from build123d import *

# Parameters (mm, degrees)
BOSS_EXTRUDE1_START            = -6.5
BOSS_EXTRUDE1_OUTLINE_W        = 7.364142843
BOSS_EXTRUDE1_OUTLINE_H        = 4.764142843
BOSS_EXTRUDE1_DEPTH            = 6.5
SKETCH2_W                      = 7.364142843
SKETCH2_H                      = 6.5
BOSS_EXTRUDE2_DEPTH            = 0.535857157
SKETCH3_W                      = 5.3
SKETCH3_H                      = 6.5
BOSS_EXTRUDE3_DEPTH            = 11.135857157
CUT_EXTRUDE1_DEPTH             = 0.7
SKETCH5_W                      = 1.14
SKETCH5_H                      = 1.5
CUT_EXTRUDE2_DEPTH             = 0.95
CUT_EXTRUDE3_DEPTH             = 0.7
SKETCH7_W                      = 1.14
SKETCH7_H                      = 1.5
CUT_EXTRUDE4_DEPTH             = 0.95
SKETCH8_W                      = 5.2
SKETCH8_H                      = 0.5
CUT_EXTRUDE5_DEPTH             = 18.075201317
CUT_EXTRUDE6_DEPTH             = 18.075201317
SKETCH10_W                     = 2
SKETCH10_H                     = 0.5
BOSS_EXTRUDE4_DEPTH            = 3.5
SKETCH11_W                     = 2
SKETCH11_H                     = 0.5
BOSS_EXTRUDE5_DEPTH            = 3.5
SKETCH12_W                     = 2
SKETCH12_H                     = 0.5
BOSS_EXTRUDE6_DEPTH            = 3.5
SKETCH13_W                     = 0.8
SKETCH13_H                     = 2.7
BOSS_EXTRUDE7_DEPTH            = 0.5
SKETCH14_W                     = 0.8
SKETCH14_H                     = 2.7
BOSS_EXTRUDE8_DEPTH            = 0.5
SKETCH15_R                     = 2.55
BOSS_EXTRUDE9_DEPTH            = 0.7
SKETCH16_R                     = 1.8
BOSS_EXTRUDE10_DEPTH           = 0.411605056
SKETCH17_R                     = 1.325
BOSS_EXTRUDE11_DEPTH           = 1
BOSS_EXTRUDE12_REACH           = 22.64
BOSS_EXTRUDE12_END_RADIUS      = 1.5
SKETCH18_R                     = 0.85
SKETCH19_R                     = 1.5
BOSS_EXTRUDE13_DEPTH           = 1.5
BOSS_EXTRUDE14_START           = 1.5
SKETCH20_R                     = 1.5
BOSS_EXTRUDE14_DEPTH           = 1.5
SKETCH21_W                     = 1.65
SKETCH21_H                     = 0.5
CUT_EXTRUDE7_DEPTH             = 1.5
SKETCH22_W                     = 1.65
SKETCH22_H                     = 0.5
CUT_EXTRUDE8_DEPTH             = 1.5
BOSS_EXTRUDE15_DEPTH           = 0.3
BOSS_EXTRUDE16_START           = 0.3
BOSS_EXTRUDE16_DEPTH           = 0.3
SKETCH25_W                     = 0.29999989
SKETCH25_H                     = 3.4
CUT_EXTRUDE9_DEPTH             = 0.5
SKETCH26_W                     = 1.8
SKETCH26_H                     = 2.5
SKETCH27_W                     = 0.3
SKETCH27_H                     = 1.5
SKETCH28_W                     = 0.3
SKETCH28_H                     = 1.5
F_1_4_1_4_DIAMETER_HOLE1_D     = 1.4
F_1_4_1_4_DIAMETER_HOLE1_DEPTH = 1.5
F_1_4_1_4_DIAMETER_HOLE2_D     = 1.4
F_1_4_1_4_DIAMETER_HOLE2_DEPTH = 1.5
FILLET1_R                      = 1.2
FILLET2_R                      = 2.5


with BuildPart() as part:
    # Boss-Extrude1: read off the stored shape, not the designer's step
    # Boss-Extrude1 outline → Boss-Extrude1 (new body)
    with BuildSketch(Plane(origin=(0, 3, 0), x_dir=(1, 0, 0), z_dir=(0, 1, 0)).offset(BOSS_EXTRUDE1_START)):
        with Locations((1.032071421, 2.917928579)):
            Rectangle(BOSS_EXTRUDE1_OUTLINE_W, BOSS_EXTRUDE1_OUTLINE_H)
    extrude(amount=BOSS_EXTRUDE1_DEPTH)

    # Boss-Extrude1 2 outline → Boss-Extrude1 2 (revolve)
    with BuildSketch(Plane(origin=(4, 0, -1.25), x_dir=(1, 0, 0), z_dir=(0, 0, 1))):
        with BuildLine():
            Line((0, 2.999999999), (0.714142844, 2.999999999))
            ThreePointArc((0.714142844, 2.999999999), (0.387298335, 3.221954446), (0, 3.3))
            Line((0, 3.3), (0, 2.999999999))
        make_face()
    revolve(axis=Axis((4, 0, -1.25), (0, 1, 0)))

    # Sketch2 → Boss-Extrude2 (add)
    with BuildSketch(Plane.XY.offset(-0.535857157)):
        with Locations((1.032071421, -0.25)):
            Rectangle(SKETCH2_W, SKETCH2_H)
    extrude(amount=BOSS_EXTRUDE2_DEPTH)

    # Sketch3 → Boss-Extrude3 (add)
    with BuildSketch(Plane(origin=(4.714142843, 0, 0), x_dir=(0, 0, -1), z_dir=(1, 0, 0))):
        with Locations((2.65, -0.25)):
            Rectangle(SKETCH3_W, SKETCH3_H)
    extrude(amount=BOSS_EXTRUDE3_DEPTH)

    # Sketch4 → Cut-Extrude1 (cut)
    with BuildSketch(Plane(origin=(9.95, 0, 0), x_dir=(0, -1, 0), z_dir=(-1, 0, 0))):
        Polygon((-1.5, -0.5), (-1.5, -1.65), (0, -1.65), (0, 0), (-3, 0), (-3, -0.5), align=None)
    extrude(amount=-CUT_EXTRUDE1_DEPTH, mode=Mode.SUBTRACT)

    # Sketch5 → Cut-Extrude2 (cut)
    with BuildSketch(Plane(origin=(9.95, 0, 0), x_dir=(0, 0, -1), z_dir=(1, 0, 0))):
        with Locations((1.08, 0.75)):
            Rectangle(SKETCH5_W, SKETCH5_H)
    extrude(amount=-CUT_EXTRUDE2_DEPTH, mode=Mode.SUBTRACT)

    # Sketch6 → Cut-Extrude3 (cut)
    with BuildSketch(Plane(origin=(9.95, 0, 0), x_dir=(0, -1, 0), z_dir=(-1, 0, 0))):
        Polygon((-3, -5.3), (0, -5.3), (0, -3.65), (-1.5, -3.65), (-1.5, -4.8), (-3, -4.8), align=None)
    extrude(amount=-CUT_EXTRUDE3_DEPTH, mode=Mode.SUBTRACT)

    # Sketch7 → Cut-Extrude4 (cut)
    with BuildSketch(Plane(origin=(9.95, 0, 0), x_dir=(0, 0, -1), z_dir=(1, 0, 0))):
        with Locations((4.22, 0.75)):
            Rectangle(SKETCH7_W, SKETCH7_H)
    extrude(amount=-CUT_EXTRUDE4_DEPTH, mode=Mode.SUBTRACT)

    # Sketch8 → Cut-Extrude5 (cut, through all)
    with BuildSketch(Plane.XY):
        with Locations((13.25, -3.25)):
            Rectangle(SKETCH8_W, SKETCH8_H)
    extrude(amount=-CUT_EXTRUDE5_DEPTH, mode=Mode.SUBTRACT)

    # Sketch9 → Cut-Extrude6 (cut, through all)
    with BuildSketch(Plane.XY):
        with BuildLine():
            Line((13.565685425, 1.55), (12.434314575, 1.55))
            ThreePointArc((12.434314575, 1.55), (11.35, 0), (12.434314575, -1.55))
            Line((12.434314575, -1.55), (13.565685425, -1.55))
            ThreePointArc((13.565685425, -1.55), (14.65, 0), (13.565685425, 1.55))
        make_face()
    extrude(amount=-CUT_EXTRUDE6_DEPTH, mode=Mode.SUBTRACT)

    # Sketch10 → Boss-Extrude4 (add)
    with BuildSketch(Plane.XZ.offset(3.5)):
        with Locations((-0.38, -2.65)):
            Rectangle(SKETCH10_W, SKETCH10_H)
    extrude(amount=BOSS_EXTRUDE4_DEPTH)

    # Sketch11 → Boss-Extrude5 (add)
    with BuildSketch(Plane.XZ.offset(3.5)):
        with Locations((4, -2.65)):
            Rectangle(SKETCH11_W, SKETCH11_H)
    extrude(amount=BOSS_EXTRUDE5_DEPTH)

    # Sketch12 → Boss-Extrude6 (add)
    with BuildSketch(Plane.XZ.offset(3.5)):
        with Locations((8.38, -2.65)):
            Rectangle(SKETCH12_W, SKETCH12_H)
    extrude(amount=BOSS_EXTRUDE6_DEPTH)

    # Sketch13 → Boss-Extrude7 (add)
    with BuildSketch(Plane.XZ.offset(3.5)):
        with Locations((1.45, -2.65)):
            Rectangle(SKETCH13_W, SKETCH13_H)
    extrude(amount=BOSS_EXTRUDE7_DEPTH)

    # Sketch14 → Boss-Extrude8 (add)
    with BuildSketch(Plane.XZ.offset(3.5)):
        with Locations((6.55, -2.65)):
            Rectangle(SKETCH14_W, SKETCH14_H)
    extrude(amount=BOSS_EXTRUDE8_DEPTH)

    # Sketch15 → Boss-Extrude9 (add)
    with BuildSketch(Plane(origin=(0, 3, 0), x_dir=(-1, 0, 0), z_dir=(0, 1, 0))):
        with Locations(Location((0, -2.65, 0), (0, 0, 90))):
            Circle(SKETCH15_R)
    extrude(amount=BOSS_EXTRUDE9_DEPTH)

    # Sketch16 → Boss-Extrude10 (add)
    with BuildSketch(Plane(origin=(0, 3.7, 0), x_dir=(-1, 0, 0), z_dir=(0, 1, 0))):
        with Locations(Location((0, -2.65, 0), (0, 0, 270))):
            Circle(SKETCH16_R)
    extrude(amount=BOSS_EXTRUDE10_DEPTH)

    # Sketch17 → Boss-Extrude11 (add)
    with BuildSketch(Plane(origin=(0, 4.111605056, 0), x_dir=(-1, 0, 0), z_dir=(0, 1, 0))):
        with Locations(Location((0, -2.65, 0), (0, 0, 90))):
            Circle(SKETCH17_R)
    extrude(amount=BOSS_EXTRUDE11_DEPTH)

    # Boss-Extrude12: up to this sphere (the profile starts inside it)
    boss_extrude12_end = Location((0, 4.811605056, -2.65)) * Sphere(BOSS_EXTRUDE12_END_RADIUS, mode=Mode.PRIVATE)
    # Sketch18 → Boss-Extrude12 (add, up to the surface)
    with BuildSketch(Plane(origin=(0, 5.111605056, 0), x_dir=(-1, 0, 0), z_dir=(0, 1, 0)), mode=Mode.PRIVATE) as boss_extrude12_sk1:
        with Locations(Location((0, -2.65, 0), (0, 0, 90))):
            Circle(SKETCH18_R)
    boss_extrude12_tool1 = extrude(boss_extrude12_sk1.sketch, amount=BOSS_EXTRUDE12_REACH, mode=Mode.PRIVATE) & boss_extrude12_end
    add(boss_extrude12_tool1.solids().sort_by_distance((0, 5.111605, -2.65))[0])

    # Sketch19 → Boss-Extrude13 (add)
    with BuildSketch(Plane.XY):
        with Locations(Location((0, 0, 0), (0, 0, 180))):
            Circle(SKETCH19_R)
    extrude(amount=BOSS_EXTRUDE13_DEPTH)

    # Sketch20 → Boss-Extrude14 (add)
    with BuildSketch(Plane(origin=(0, 0, -5.3), x_dir=(-1, 0, 0), z_dir=(0, 0, -1)).offset(BOSS_EXTRUDE14_START)):
        Circle(SKETCH20_R)
    extrude(amount=-BOSS_EXTRUDE14_DEPTH)

    # Sketch21 → Cut-Extrude7 (cut)
    with BuildSketch(Plane(origin=(0, 3, 0), x_dir=(-1, 0, 0), z_dir=(0, 1, 0))):
        with Locations((-9.125, -0.25)):
            Rectangle(SKETCH21_W, SKETCH21_H)
    extrude(amount=-CUT_EXTRUDE7_DEPTH, mode=Mode.SUBTRACT)

    # Sketch22 → Cut-Extrude8 (cut)
    with BuildSketch(Plane(origin=(0, 3, 0), x_dir=(-1, 0, 0), z_dir=(0, 1, 0))):
        with Locations((-9.125, -5.05)):
            Rectangle(SKETCH22_W, SKETCH22_H)
    extrude(amount=-CUT_EXTRUDE8_DEPTH, mode=Mode.SUBTRACT)

    # Sketch23 → Boss-Extrude15 (add)
    with BuildSketch(Plane.XY.offset(-0.5)):
        with BuildLine():
            Line((9.052786405, 3), (9.947213595, 3))
            ThreePointArc((9.947213595, 3), (9.5, 2), (9.052786405, 3))
        make_face()
    extrude(amount=BOSS_EXTRUDE15_DEPTH)

    # Sketch24 → Boss-Extrude16 (add)
    with BuildSketch(Plane(origin=(0, 0, -4.8), x_dir=(-1, 0, 0), z_dir=(0, 0, -1)).offset(BOSS_EXTRUDE16_START)):
        with BuildLine():
            Line((-9.947213595, 3), (-9.052786405, 3))
            ThreePointArc((-9.052786405, 3), (-9.5, 2), (-9.947213595, 3))
        make_face()
    extrude(amount=-BOSS_EXTRUDE16_DEPTH)

    # Sketch25 → Cut-Extrude9 (cut)
    with BuildSketch(Plane(origin=(0, 3, 0), x_dir=(-1, 0, 0), z_dir=(0, 1, 0))):
        with Locations((-10.149999945, -2.65)):
            Rectangle(SKETCH25_W, SKETCH25_H)
    extrude(amount=-CUT_EXTRUDE9_DEPTH, mode=Mode.SUBTRACT)

    # Sketch26 → Cut-Revolve1 (revolve, cut)
    with BuildSketch(Plane(origin=(0, 0, -2.65), x_dir=(-1, 0, 0), z_dir=(0, 0, -1))):
        with Locations((-0.9, 1.75)):
            Rectangle(SKETCH26_W, SKETCH26_H)
    revolve(axis=Axis((0, 0.5, -2.65), (0, 1, 0)), mode=Mode.SUBTRACT)

    # Sketch27 → Revolve1 (revolve)
    with BuildSketch(Plane.XY.offset(-4.45), mode=Mode.PRIVATE) as revolve1_sk:
        with Locations((10.1, 0.75)):
            Rectangle(SKETCH27_W, SKETCH27_H)
    revolve(revolve1_sk.sketch.rotate(Axis((9.95, 1.5, -4.45), (0, -1, 0)), 270), axis=Axis((9.95, 1.5, -4.45), (0, -1, 0)))

    # Sketch28 → Revolve2 (revolve)
    with BuildSketch(Plane.XY.offset(-0.85), mode=Mode.PRIVATE) as revolve2_sk:
        with Locations((10.1, 0.75)):
            Rectangle(SKETCH28_W, SKETCH28_H)
    revolve(revolve2_sk.sketch.rotate(Axis((9.95, 1.5, -0.85), (0, -1, 0)), 270), axis=Axis((9.95, 1.5, -0.85), (0, -1, 0)))

    # Ø1.4 (1.4) Diameter Hole1
    with Locations(Plane(origin=(0, 0, -6.8), x_dir=(-1, 0, 0), z_dir=(0, 0, -1))):
        with Locations((0.093266982, 0)):
            Hole(F_1_4_1_4_DIAMETER_HOLE1_D / 2, depth=F_1_4_1_4_DIAMETER_HOLE1_DEPTH)

    # Ø1.4 (1.4) Diameter Hole2
    with Locations(Plane.XY.offset(1.5)):
        with Locations((0, 0)):
            Hole(F_1_4_1_4_DIAMETER_HOLE2_D / 2, depth=F_1_4_1_4_DIAMETER_HOLE2_DEPTH)

    # Fillet1
    fillet1_edges = [part.edges().sort_by_distance(p)[0] for p in [
        (8.3, 1.5, -0.25),
        (8.3, 1.5, -5.05),
    ]]
    fillet(fillet1_edges, radius=FILLET1_R)

    # Fillet2
    fillet2_edges = [part.edges().sort_by_distance(p)[0] for p in [
        (15.85, 3, -2.65),
        (15.85, -3, -2.65),
    ]]
    fillet(fillet2_edges, radius=FILLET2_R)


solid = part.part
Design review of the part built by this model. Coordinates are the model's own, in mm. A direction names the side the tool comes from. Coordinates: 2 decimals unless noted, no trailing zeros. Order: outer loops, then holes, each group sorted by start corner. A loop starts at its lowest first (then second) coordinate and runs counter-clockwise, first axis right, second up. Notation, with made-up numbers: (-25, 81) -> (11, 81) arc R15 ccw to (11, 99) -> close; hole circle Ø4 at (42.25, 45). An arc over 180 degrees is marked (long way). One line per item, written item: value.
1) Draft analysis for pull direction Y (two halves, no side actions). For faces 1 (the face through (0, -5, -2.9)), 2 (the face through (12, -3, -3)), 3 (the face through (2, 3.7, -2)), 4 (the face through (13, 1.55, -3)), state which applies: +Y half, -Y half, draft (parallel to the pull), parting line (faces both ways), or undercut.
Output values:
face 1: draft
face 2: -Y half
face 3: +Y half
face 4: undercut
2) To check wall thickness, follow probe 1 along Z at (x, y) = (0, 1.3); probe 2 along Y at (x, z) = (8, -1.75); probe 3 along Z at (x, y) = (6.25, -0.75). State the ranges of each line that lie inside material, in increasing order. Write a range as [from, to].
Output values:
probe 1: z = [-6.8, -4.45], [-0.85, 1.5]
probe 2: y = [-3.5, 3]
probe 3: z = [-5.3, 0]
3) We need section A-A, the plane y = -4.25. Give the boundary of the cut face in (x, z).
Output values:
outline: (-1.38, -2.9) -> (0.62, -2.9) -> (0.62, -2.4) -> (-1.38, -2.4) -> close; (3, -2.9) -> (5, -2.9) -> (5, -2.4) -> (3, -2.4) -> close; (7.38, -2.9) -> (9.38, -2.9) -> (9.38, -2.4) -> (7.38, -2.4) -> close
4) We need section C-C, the plane z = -5.5. Give the boundary of the cut face in (x, y).
Output values:
outline: circle Ø3 at (0, 0); hole circle Ø1.4 at (-0.09, 0)
5) We need section D-D, the plane x = 3.5. Give the boundary of the cut face in (y, z).
Output values:
outline: (-7, -2.9) -> (-3.5, -2.9) -> (-3.5, -5.3) -> (3, -5.3) -> (3, -1.76) arc R0.87 ccw to (3, -0.74) -> (3, 0) -> (-3.5, 0) -> (-3.5, -2.4) -> (-7, -2.4) -> close
6) Machinability: for faces 5 (the face through (9.6, 1.5, -1.2)), 6 (the face through (0, 0, -5.3)), 7 (the face through (0, 4.112, -1)), 8 (the face through (15.85, 0, -3)), which of the approach directions +Z, -Z, +X, -X, +Y, -Y give a long, thin tool a straight path to every point of the face, cutting with its end or side? Answer none if there is none.
Output values:
face 5: none
face 6: -Z
face 7: +Y
face 8: +Z, -Z, +X, +Y, -Y
7) We need section B-B, the plane y = -1. Give the boundary of the cut face in (x, z), then the cut area to 3 significant figures.
Output values:
outline: (-2.65, -5.3) -> (-1.12, -5.3) -> (-1.12, -6.8) -> (1.12, -6.8) -> (1.12, -5.3) -> (11.69, -5.3) -> (11.69, 0) -> (1.12, 0) -> (1.12, 1.5) -> (-1.12, 1.5) -> (-1.12, 0) -> (-2.65, 0) -> close; (14.31, -5.3) -> (15.8, -5.3) -> (15.8, 0) -> (14.31, 0) -> close
area: 90.6 mm2
8) Clearance check with flat-ended pins moving along their axes: P1, Ø7, axis at x = 10.5, y = -1.5, coming from the +Z side; P2, Ø2.5, axis at x = 1.5, z = -2, coming from the -Y side; P3, Ø4, axis at x = 8.5, y = 0.5, coming from the -Z side; P4, Ø0.8, axis at x = 9.5, z = -0.5, coming from the +Y side. State where each tip first meets the part, or that it passes through.
Output values:
P1: stops at z = 0
P2: stops at y = -7
P3: stops at z = -5.3
P4: stops at y = 3
